Build history of the part. All positions in model axes, mm. A direction names the side the tool comes from. Coordinates: 2 decimals unless noted, no trailing zeros. Write each loop counter-clockwise with the first axis right and the second up, starting at its lowest first coordinate (ties: lowest second). Pieces come first, ordered by that corner, then holes.
```python
from build123d import *

# Parameters (mm, degrees)
SKIZZE1_R                       = 18.7
SKIZZE1_R_2                     = 6.1
SKIZZE1_R_3                     = 1.75
AUFSATZ_LINEAR_AUSTRAGEN1_DEPTH = 6
SKIZZE3_R                       = 20.7
SKIZZE3_R_2                     = 18.7
AUFSATZ_LINEAR_AUSTRAGEN2_DEPTH = 27.8
AUFSATZ_LINEAR_AUSTRAGEN3_DEPTH = 21
SKIZZE7_R                       = 2.25
SCHNITT_LINEAR_AUSTRAGEN1_DEPTH = 64.928084722
SKIZZE8_R                       = 5
SCHNITT_LINEAR_AUSTRAGEN2_DEPTH = 10.5
FORMSCHR_GE1_ANGLE              = 1.5
SKIZZE9_R                       = 2.774707021
SKIZZE9_R_2                     = 1.75
SCHNITT_LINEAR_AUSTRAGEN3_DEPTH = 1.5
SKIZZE10_W                      = 19.3
SKIZZE10_H                      = 20.7
SCHNITT_LINEAR_AUSTRAGEN4_DEPTH = 50.69396358


with BuildPart() as part:
    # Skizze1 → Aufsatz-Linear austragen1 (new body)
    with BuildSketch(Plane.XY):
        Circle(SKIZZE1_R)
        with Locations((0, -7)):
            Circle(SKIZZE1_R_2, mode=Mode.SUBTRACT)
        with Locations((-7.65, 13.250188678)):
            Circle(SKIZZE1_R_3, mode=Mode.SUBTRACT)
        with Locations(Location((7.65, 13.250188678, 0), (0, 0, 180))):
            Circle(SKIZZE1_R_3, mode=Mode.SUBTRACT)
        with Locations((-15.3, 0)):
            Circle(SKIZZE1_R_3, mode=Mode.SUBTRACT)
        with Locations(Location((15.3, 0, 0), (0, 0, 180))):
            Circle(SKIZZE1_R_3, mode=Mode.SUBTRACT)
        with Locations(Location((-7.65, -13.250188678, 0), (0, 0, 180))):
            Circle(SKIZZE1_R_3, mode=Mode.SUBTRACT)
        with Locations((7.65, -13.250188678)):
            Circle(SKIZZE1_R_3, mode=Mode.SUBTRACT)
    extrude(amount=AUFSATZ_LINEAR_AUSTRAGEN1_DEPTH)

    # Skizze3 → Aufsatz-Linear austragen2 (add)
    with BuildSketch(Plane(origin=(0, 0, 0), x_dir=(-1, 0, 0), z_dir=(0, 0, -1))):
        Circle(SKIZZE3_R)
        Circle(SKIZZE3_R_2, mode=Mode.SUBTRACT)
    extrude(amount=-AUFSATZ_LINEAR_AUSTRAGEN2_DEPTH)

    # Skizze4 → Aufsatz-Linear austragen3 (add)
    with BuildSketch(Plane(origin=(0, 0, 0), x_dir=(-1, 0, 0), z_dir=(0, 0, -1))):
        with BuildLine():
            add(Edge.make_bspline(
                [(-20.7, 0), (-20.7, -18.7), (-40, -18.7)],
                knots=[0, 0, 0, 1, 1, 1], degree=2))
            Line((-40, -18.7), (-40, -20.7))
            Line((-40, -20.7), (9.3e-08, -20.7))
            ThreePointArc((9.3e-08, -20.7), (-14.637110338, -14.637110404), (-20.7, 0))
        make_face()
        with BuildLine():
            ThreePointArc((20.7, 0), (14.637110404, -14.637110338), (9.3e-08, -20.7))
            Line((9.3e-08, -20.7), (40, -20.7))
            Line((40, -20.7), (40, -18.7))
            add(Edge.make_bspline(
                [(20.7, 0), (20.7, -18.7), (40, -18.7)],
                knots=[0, 0, 0, 1, 1, 1], degree=2))
        make_face()
    extrude(amount=-AUFSATZ_LINEAR_AUSTRAGEN3_DEPTH)

    # Skizze7 → Schnitt-Linear austragen1 (cut, through all)
    with BuildSketch(Plane.XZ.offset(20.7)):
        with Locations((-34, 10.5)):
            Circle(SKIZZE7_R)
        with Locations((34, 10.5)):
            Circle(SKIZZE7_R)
    extrude(amount=-SCHNITT_LINEAR_AUSTRAGEN1_DEPTH, mode=Mode.SUBTRACT)

    # Skizze8 → Schnitt-Linear austragen2 (cut)
    with BuildSketch(Plane.XZ.offset(18.7)):
        with Locations((-34, 10.5)):
            Circle(SKIZZE8_R)
        with Locations((34, 10.5)):
            Circle(SKIZZE8_R)
    extrude(amount=-SCHNITT_LINEAR_AUSTRAGEN2_DEPTH, mode=Mode.SUBTRACT)

    # Formschr_ge1
    formschr_ge1_faces = [part.faces().sort_by_distance(p)[0] for p in [
        (18.7, 0, 16.9),
    ]]
    draft(formschr_ge1_faces, Plane.XY.offset(6), FORMSCHR_GE1_ANGLE)

    # Skizze9 → Schnitt-Linear austragen3 (cut)
    # profile 1 of 6: a face of its own
    with BuildSketch(Plane(origin=(0, 0, 0), x_dir=(-1, 0, 0), z_dir=(0, 0, -1))):
        with Locations((-7.65, 13.250188678)):
            Circle(SKIZZE9_R)
        with Locations((-7.65, 13.250188678)):
            Circle(SKIZZE9_R_2, mode=Mode.SUBTRACT)
    # profile 2 of 6: a face of its own
    with BuildSketch(Plane(origin=(0, 0, 0), x_dir=(-1, 0, 0), z_dir=(0, 0, -1))):
        with Locations(Location((7.65, 13.250188678, 0), (0, 0, 180))):
            Circle(SKIZZE9_R)
        with Locations(Location((7.65, 13.250188678, 0), (0, 0, 180))):
            Circle(SKIZZE9_R_2, mode=Mode.SUBTRACT)
    # profile 3 of 6: a face of its own
    with BuildSketch(Plane(origin=(0, 0, 0), x_dir=(-1, 0, 0), z_dir=(0, 0, -1))):
        with Locations((-15.3, 0)):
            Circle(SKIZZE9_R)
        with Locations((-15.3, 0)):
            Circle(SKIZZE9_R_2, mode=Mode.SUBTRACT)
    # profile 4 of 6: a face of its own
    with BuildSketch(Plane(origin=(0, 0, 0), x_dir=(-1, 0, 0), z_dir=(0, 0, -1))):
        with Locations(Location((15.3, 0, 0), (0, 0, 180))):
            Circle(SKIZZE9_R)
        with Locations(Location((15.3, 0, 0), (0, 0, 180))):
            Circle(SKIZZE9_R_2, mode=Mode.SUBTRACT)
    # profile 5 of 6: a face of its own
    with BuildSketch(Plane(origin=(0, 0, 0), x_dir=(-1, 0, 0), z_dir=(0, 0, -1))):
        with Locations((7.65, -13.250188678)):
            Circle(SKIZZE9_R)
        with Locations((7.65, -13.250188678)):
            Circle(SKIZZE9_R_2, mode=Mode.SUBTRACT)
    # profile 6 of 6: a face of its own
    with BuildSketch(Plane(origin=(0, 0, 0), x_dir=(-1, 0, 0), z_dir=(0, 0, -1))):
        with Locations(Location((-7.65, -13.250188678, 0), (0, 0, 180))):
            Circle(SKIZZE9_R)
        with Locations(Location((-7.65, -13.250188678, 0), (0, 0, 180))):
            Circle(SKIZZE9_R_2, mode=Mode.SUBTRACT)
    extrude(amount=-SCHNITT_LINEAR_AUSTRAGEN3_DEPTH, mode=Mode.SUBTRACT)

    # Skizze10 → Schnitt-Linear austragen4 (cut, through all)
    with BuildSketch(Plane.XY.offset(21)):
        with Locations((30.35, -10.35)):
            Rectangle(SKIZZE10_W, SKIZZE10_H)
    extrude(amount=-SCHNITT_LINEAR_AUSTRAGEN4_DEPTH, mode=Mode.SUBTRACT)


solid = part.part
```
1. Probe line 1 along Y through (x, z) = (7.65, 0.45); line 2 along Y through (x, z) = (-7, 5) (1 decimal); line 3 along Z through (x, y) = (-34, -19). List the from-to ranges inside material, lowest first.
Computed values:
line 1: y = -20.7 to -16.02, -10.48 to 10.48, 16.02 to 19.23
line 2: y = -20.7 to -14.9, -11.6 to 11.6, 14.9 to 19.5
line 3: z = 0 to 8.25, 12.75 to 21
2. 3-axis set-ups, long thin cutter, end or side, ignore diameter. For faces 4 (the face through (-4.84, -10.71, 2.96)), 5 (the face through (-21, -17, 21)), 6 (the face through (8, -11, 1.5)), 7 (the face through (-10.2, 16.01, 16.75)), 8 (the face through (-14, -14, 27.8)): which of +Z, -Z, +X, -X, +Y, -Y reach the whole face in a straight line?
Computed values:
face 4: +Z, -Z
face 5: +Z, -X, -Y
face 6: -Z
face 7: +Z
face 8: +Z, +X, -X, +Y, -Y
3. Mould opens along Z. For faces 1 (the face through (-2, 0, 0)), 2 (the face through (-32, -18.7, 9)), 3 (the face through (9.039, 14.315, 3.718)) say: +Z half, -Z half, draft (parallel to the pull), parting line (faces both ways), or undercut.
Computed values:
face 1: -Z half
face 2: undercut
face 3: draft
4. Saw through at D-D on x = -20. List the corners of the cut face in (y, z), plus the area to 3 significant figures.
Computed values:
outline: (-20.7, 0) - (5.34, 0) - (5.34, 27.8) - (-5.34, 27.8) - (-5.34, 21) - (-20.7, 21) - close
area: 619 mm2
5. Saw through at A-A on z = 9. State how many separate pieces and enclosed holes the cut face has, plus the area to 3 significant figures.
Computed values:
separate pieces: 2
enclosed holes: 1
area: 507 mm2
6. Flat gauge pins, fed straight in: pin 1 (12 mm diameter, centred on x = -31.5, y = -13.5, fed in from +Z); pin 2 (4 mm diameter, centred on x = 7.65, y = 13.25, fed in from +Z); pin 3 (6 mm diameter, centred on x = -25.5, y = -8.5, fed in from +Z); pin 4 (4.5 mm diameter, centred on x = 7.65, y = -13.25, fed in from -Z). Where does each tip first touch, or does it go through?
Computed values:
pin 1: stops at z = 21
pin 2: stops at z = 6
pin 3: passes through
pin 4: stops at z = 1.5
